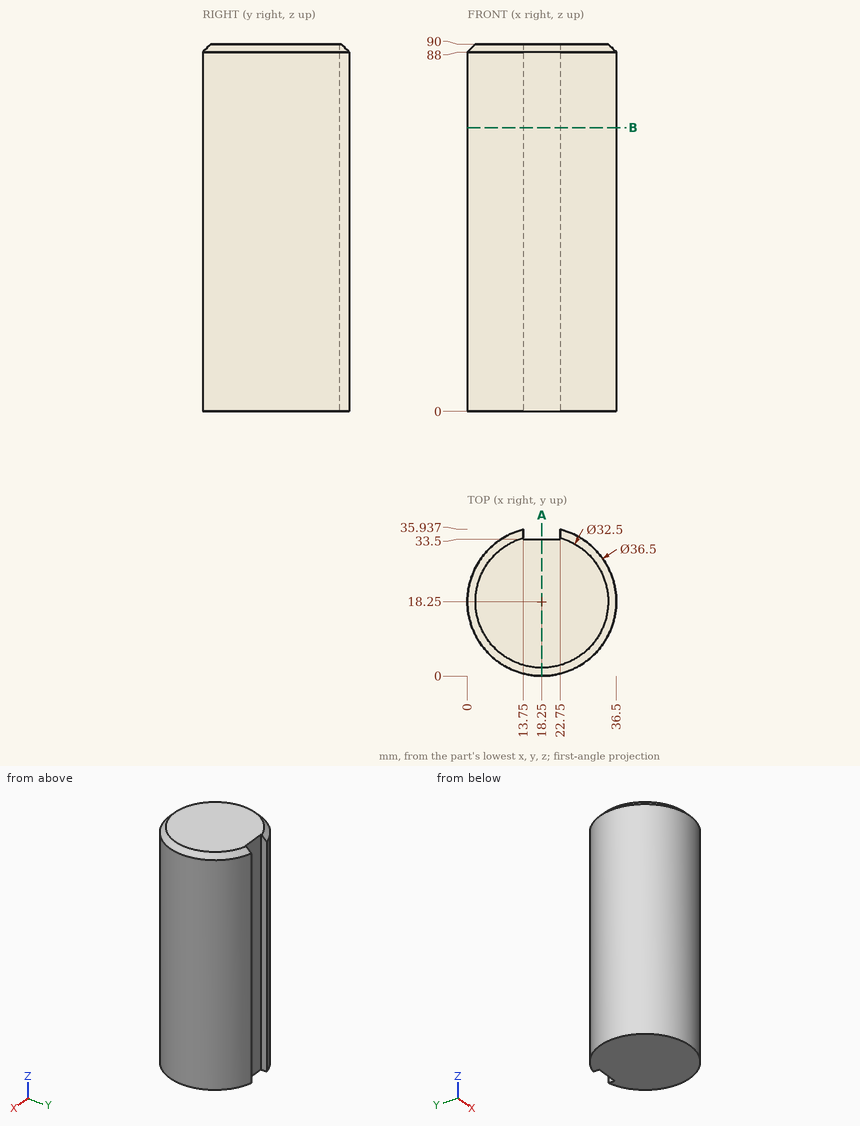
Geometry: see drawing. Coordinates: mm, zero at the bounding-box minimum. Round coordinates to 2 decimals unless told otherwise and drop trailing zeros. Loops run counter-clockwise (first coordinate to the right, second up) from the corner with the lowest first, then second, coordinate; pieces in that order, holes last. Notation, with made-up numbers: (41, -26.75) - (73, -26.75) arc R15 cw to (73, -1.75) - close; hole circle Ø2 at (-37, 64.5). An arc over 180 degrees is marked (long way). Write item = value, one per line. Start each with the question number.
(1) Pin query (flat end, axial travel): pin 1 (5 mm diameter, centred on x = 32, z = 75, fed in from -Y); pin 2 (3 mm diameter, centred on x = 4.5, z = 25, fed in from -Y); pin 3 (0.7 mm diameter, centred on y = 35, z = 43, fed in from -X) (1 decimal); pin 4 (6 mm diameter, centred on x = 18, y = 8.5, fed in from -Z). Return the tip coordinate at first contact, or that it passes through.
(2) Section query A-A, the plane x = 18.25. Output: boundary loops of the cut face in (y, z).
(3) Section query B-B, the plane z = 69.5. Output: boundary loops of the cut face in (x, y), plus the area to 3 significant figures.
(4) Ray query, line 1 along X through (y, z) = (18, 65.5); line 2 along Y through (x, z) = (18.5, 38.5); line 3 along X through (y, z) = (21, 34). Return the intervals inside material, ascending. Write a range as from..to.
Conclusion:
q1.pin_1 = 3.88
q1.pin_2 = 4.72
q1.pin_3 = 10.2
q1.pin_4 = 0
q2.outline = (0, 0) - (33.5, 0) - (33.5, 90) - (2, 90) - (0, 88) - close
q3.outline = (13.75, 33.5) - (13.75, 35.94) arc R18.25 ccw (long way) to (22.75, 35.94) - (22.75, 33.5) - close
q3.area = 1,020 mm2
q4.line_1 = 0..36.5
q4.line_2 = 0..33.5
q4.line_3 = 0.21..36.29
